```python
from build123d import *

# Parameters (mm, degrees)
SKETCH1_W           = 30
SKETCH1_H           = 30
SKETCH1_W_2         = 20.5
SKETCH1_H_2         = 20.5
BOSS_EXTRUDE1_DEPTH = 20
SKETCH2_W           = 30
SKETCH2_H           = 30
BOSS_EXTRUDE3_DEPTH = 10
SKETCH4_W           = 1.5
SKETCH4_H           = 3.5
CUT_REVOLVE1_ANGLE  = 180
SKETCH5_W           = 14.323407416
SKETCH5_H           = 3.5
CUT_EXTRUDE2_DEPTH  = 1.5
SKETCH6_W           = 20.5
SKETCH6_H           = 20.5
CUT_EXTRUDE3_DEPTH  = 2


with BuildPart() as part:
    # Sketch1 → Boss-Extrude1 (new body)
    with BuildSketch(Plane.XY):
        Rectangle(SKETCH1_W, SKETCH1_H)
        Rectangle(SKETCH1_W_2, SKETCH1_H_2, mode=Mode.SUBTRACT)
    extrude(amount=BOSS_EXTRUDE1_DEPTH)

    # Sketch2 → Boss-Extrude3 (add)
    with BuildSketch(Plane(origin=(0, 0, 0), x_dir=(-1, 0, 0), z_dir=(0, 0, -1))):
        Rectangle(SKETCH2_W, SKETCH2_H)
    extrude(amount=BOSS_EXTRUDE3_DEPTH)

    # Sketch4 → Cut-Revolve1 (revolve, cut)
    with BuildSketch(Plane(origin=(0, 0, -10), x_dir=(-1, 0, 0), z_dir=(0, 0, -1))):
        Polygon((0, 0), (0, 15), (7.8, 15), (7.8, 8.75), (7.8, 7.65), (7.8, 0), align=None)
        with Locations((11.55, 8.2)):
            Rectangle(SKETCH4_W, SKETCH4_H)
    cut_revolve1 = revolve(axis=Axis((0, 0, -10), (0, 1, 0)), revolution_arc=CUT_REVOLVE1_ANGLE, mode=Mode.SUBTRACT)

    # Sketch5 → Cut-Extrude2 (cut)
    with BuildSketch(Plane.XY):
        with Locations((0, 8.2)):
            Rectangle(SKETCH5_W, SKETCH5_H)
    cut_extrude2 = extrude(amount=-CUT_EXTRUDE2_DEPTH, mode=Mode.SUBTRACT)

    # Mirror1: Cut-Revolve1, Cut-Extrude2 across plane
    add(cut_revolve1.mirror(Plane(origin=(0, 0, -10), x_dir=(0, 0, 1), z_dir=(0, -1, 0))), mode=Mode.SUBTRACT)
    add(cut_extrude2.mirror(Plane(origin=(0, 0, -10), x_dir=(0, 0, 1), z_dir=(0, -1, 0))), mode=Mode.SUBTRACT)

    # Sketch6 → Cut-Extrude3 (cut)
    with BuildSketch(Plane.XY):
        Rectangle(SKETCH6_W, SKETCH6_H)
    extrude(amount=-CUT_EXTRUDE3_DEPTH, mode=Mode.SUBTRACT)


solid = part.part
```
Part model, mm, in its own coordinate system. A direction names the side the tool comes from. Round coordinates to 2 decimals unless told otherwise and drop trailing zeros. Loops run counter-clockwise (first coordinate to the right, second up) from the corner with the lowest first, then second, coordinate; pieces in that order, holes last. Notation, with made-up numbers: (83.5, -23) -> (116.5, -23) arc R8 cw to (116.5, -18) -> close; hole circle Ø11 at (-21, 51.25). An arc over 180 degrees is marked (long way). Use one line per item in the form item = value. Start each with the question number.
Item 1: Two-plate mould, pull along Y, no slides. Class faces 1 (the cylindrical face through (11.516, 8.224, -5.678)), 2 (the flat face through (0, -15, 5)), 3 (the flat face through (-11, 6.45, -6)), 4 (the flat face through (11, 0, -10)): released by +Y, released by -Y, zero draft, split by the parting line, or undercut.
Item 2: Tool access for faces 5 (the cylindrical face through (9.85, -8.22, -5.57)), 6 (the cylindrical face through (-0.17, 0.21, -2.2)), 7 (the flat face through (0, 0, -2)): list every direction of +Z, -Z, +X, -X, +Y, -Y with a clear straight run to the whole face (end or side of a thin tool).
Item 3: Drill centre lines: line 1 along X through (y, z) = (6, 13.25); line 2 along X through (y, z) = (-9.75, -3). Where is each one in solid material? Low to high.
Item 4: Drop a flat-ended pin along its axis: pin 1 Ø10 at (x, y) = (-5, -0.5) entering from +Z. Give the stop position or say it passes through.
Item 5: Band-saw the part on A-A (z = -3.5). List the corners of the cut face in (x, y).
Item 6: Band-saw the part on B-B (z = 16.5). List the corners of the cut face in (x, y).
Item 7: Band-saw the part on D-D (y = 3.5). List the corners of the cut face in (x, z).
Item 8: Band-saw the part on C-C (x = 0). List the corners of the cut face in (y, z), plus the area to 3 significant figures.
Data:
q1.face_1 = undercut
q1.face_2 = released by -Y
q1.face_3 = undercut
q1.face_4 = zero draft
q2.face_5 = none
q2.face_6 = -Z, +Y, -Y
q2.face_7 = +Z
q3.line_1 = -15 to -10.25, 10.25 to 15
q3.line_2 = -15 to -10.11, -8.22 to -3.44, 3.44 to 8.22, 10.11 to 15
q4.pin_1 = -2
q5.outline = (-15, -15) -> (-4.31, -15) -> (-4.31, 15) -> (-15, 15) -> close; (4.31, -15) -> (15, -15) -> (15, 15) -> (4.31, 15) -> close; hole (-10.44, -9.95) -> (-8.62, -9.95) -> (-8.62, -6.45) -> (-10.44, -6.45) -> close; hole (-10.44, 6.45) -> (-8.62, 6.45) -> (-8.62, 9.95) -> (-10.44, 9.95) -> close; hole (8.62, -9.95) -> (10.44, -9.95) -> (10.44, -6.45) -> (8.62, -6.45) -> close; hole (8.62, 6.45) -> (10.44, 6.45) -> (10.44, 9.95) -> (8.62, 9.95) -> close
q6.outline = (-15, -15) -> (15, -15) -> (15, 15) -> (-15, 15) -> close; hole (-10.25, -10.25) -> (10.25, -10.25) -> (10.25, 10.25) -> (-10.25, 10.25) -> close
q7.outline = (-15, -10) -> (-7.8, -10) arc R7.8 cw to (7.8, -10) -> (15, -10) -> (15, 20) -> (10.25, 20) -> (10.25, -2) -> (-10.25, -2) -> (-10.25, 20) -> (-15, 20) -> close
q8.outline = (-15, -2.2) -> (15, -2.2) -> (15, 20) -> (10.25, 20) -> (10.25, -2) -> (-10.25, -2) -> (-10.25, 20) -> (-15, 20) -> close
q8.area = 215 mm^2
